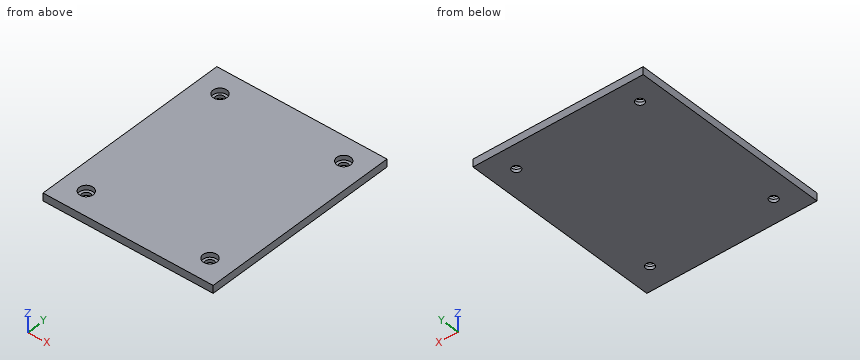
from build123d import *

# Parameters (mm, degrees)
SKETCH1_W           = 130
SKETCH1_H           = 110
BOSS_EXTRUDE1_DEPTH = 5
SKETCH3_R           = 2.75
CUT_EXTRUDE1_DEPTH  = 86.293610546
SKETCH4_R           = 4.5
CUT_EXTRUDE2_DEPTH  = 3


with BuildPart() as part:
    # Sketch1 → Boss-Extrude1 (new body)
    with BuildSketch(Plane(origin=(0, 0, 0), x_dir=(0, 1, 0), z_dir=(0, 0, 1))):
        Rectangle(SKETCH1_W, SKETCH1_H)
    extrude(amount=BOSS_EXTRUDE1_DEPTH)

    # Sketch3 → Cut-Extrude1 (cut, through all)
    with BuildSketch(Plane.XY.offset(5)):
        with Locations((-40, 50)):
            Circle(SKETCH3_R)
        with Locations((40, -50)):
            Circle(SKETCH3_R)
        with Locations((-40, -50)):
            Circle(SKETCH3_R)
        with Locations((40, 50)):
            Circle(SKETCH3_R)
    extrude(amount=-CUT_EXTRUDE1_DEPTH, mode=Mode.SUBTRACT)

    # Sketch4 → Cut-Extrude2 (cut)
    with BuildSketch(Plane.XY.offset(5)):
        with Locations((-40, 50)):
            Circle(SKETCH4_R)
        with Locations((40, 50)):
            Circle(SKETCH4_R)
        with Locations((40, -50)):
            Circle(SKETCH4_R)
        with Locations((-40, -50)):
            Circle(SKETCH4_R)
    extrude(amount=-CUT_EXTRUDE2_DEPTH, mode=Mode.SUBTRACT)


solid = part.part
Source: CAD feature listing. Evaluate the final solid. Frame: model axes, mm. Coordinates: 2 decimals unless noted, no trailing zeros. Order: outer loops, then holes, each group sorted by start corner. A loop starts at its lowest first (then second) coordinate and runs counter-clockwise, first axis right, second up.
Item 1: First-contact query: P1, Ø7, axis at x = -40, y = 50, coming from the +Z side. Flat tip, straight axial feed; report the tip coordinate or a pass-through.
Output values:
P1: stops at z = 2
Item 2: Material intervals for line 1 (Y direction, x = 40, z = 3.2); line 2 (Y direction, x = 40, z = 1.5); line 3 (X direction, y = 49, z = 4.35), sorted ascending.
Output values:
line 1: y = -65 to -54.5, -45.5 to 45.5, 54.5 to 65
line 2: y = -65 to -52.75, -47.25 to 47.25, 52.75 to 65
line 3: x = -55 to -44.39, -35.61 to 35.61, 44.39 to 55
Item 3: Cut plane B-B (x = -40). Return loops of the section in (y, z), plus the area to 3 significant figures.
Output values:
outline: (-65, 0) - (-52.75, 0) - (-52.75, 2) - (-54.5, 2) - (-54.5, 5) - (-65, 5) - close; (-47.25, 0) - (47.25, 0) - (47.25, 2) - (45.5, 2) - (45.5, 5) - (-45.5, 5) - (-45.5, 2) - (-47.25, 2) - close; (52.75, 0) - (65, 0) - (65, 5) - (54.5, 5) - (54.5, 2) - (52.75, 2) - close
area: 574 mm2
Item 4: Cut plane C-C (z = 3.2). Return loops of the section in (x, y), plus the area to 3 significant figures.
Output values:
outline: (-55, -65) - (55, -65) - (55, 65) - (-55, 65) - close; hole circle Ø9 at (-40, -50); hole circle Ø9 at (-40, 50); hole circle Ø9 at (40, -50); hole circle Ø9 at (40, 50)
area: 14,000 mm2
Item 5: Cut plane A-A (y = 50). Return loops of the section in (x, z), plus the area to 3 significant figures.
Output values:
outline: (-55, 0) - (-42.75, 0) - (-42.75, 2) - (-44.5, 2) - (-44.5, 5) - (-55, 5) - close; (-37.25, 0) - (37.25, 0) - (37.25, 2) - (35.5, 2) - (35.5, 5) - (-35.5, 5) - (-35.5, 2) - (-37.25, 2) - close; (42.75, 0) - (55, 0) - (55, 5) - (44.5, 5) - (44.5, 2) - (42.75, 2) - close
area: 474 mm2
